Autodesk Inventor part; units mm, degrees
ref_plane "YZ Plane" through (0, 0, 0) normal (1, 0, 0) x (0, 1, 0)
ref_plane "XZ Plane" through (0, 0, 0) normal (0, 1, 0) x (-1, 0, 0)
ref_plane "XY Plane" through (0, 0, 0) normal (0, 0, 1) x (1, 0, 0)
sketch "Sketch1" plane through (0, 0, 0) normal (1, 0, 0) x (0, 1, 0)
  line L0 (0, 0) -> (60, 0)
  line L1 (60, 0) -> (60, 20)
  line L2 (60, 20) -> (0, 20)
  line L3 (0, 20) -> (0, 0)
  line L4 (60, 10) -> (0, 10) construction
  line L5 (60, 10) -> (30, 10) construction
  line L6 (30, 10) -> (0, 10) construction
  circle A0 centre (45, 10) radius 2.75
  circle A1 centre (15, 10) radius 2.75
  dimension "d0" = 60
  dimension "d1" = 20
  dimension "d2" = 5.5
  dimension "d3" = 5.5
extrude "Extrusion1" add sketch "Sketch1" against normal blind 6
sketch "Sketch2" plane through (-6, 0, 0) normal (-1, 0, 0) x (0, 0, 1)
  circle A0 centre (10, 45) radius 2.75
  circle A1 centre (10, 15) radius 2.75
  circle A2 centre (10, 45) radius 6.25
  circle A3 centre (10, 15) radius 6.25
  line L0 (20, 60) -> (0, 60)
  line L1 (12, 60) -> (12, 0)
  line L2 (8, 60) -> (8, 0)
  line L3 (0, 0) -> (20, 0)
  line L4 (0, 60) -> (0, 0)
  line L5 (20, 0) -> (20, 60)
  line L6 (12, 56.5) -> (17, 56.5)
  line L7 (17, 56.5) -> (17, 60)
  line L8 (8, 56.5) -> (3, 56.5)
  line L9 (3, 56.5) -> (3, 60)
  line L10 (8, 3.5) -> (3, 3.5)
  line L11 (3, 3.5) -> (3, 0)
  line L12 (12, 3.5) -> (17, 3.5)
  line L13 (17, 3.5) -> (17, 0)
  point P0 (12, 39.0786)
  point P1 (12, 50.9214)
  point P2 (8, 50.9214)
  point P3 (8, 39.0786)
  point P4 (8, 20.9214)
  point P5 (8, 9.0786)
  point P6 (12, 9.0786)
  point P7 (12, 20.9214)
  dimension "d6" = 3.5
  dimension "d7" = 8
  dimension "d8" = 8
  dimension "d9" = 3.5
  dimension "d10" = 3.5
  dimension "d11" = 3.5
  dimension "d16" = 3.5
extrude "Extrusion2" add sketch "Sketch2" along normal blind 22.1 contours A0 L1 A2 | A0 L2 A2 L1 | L1 A2 L2 A0 | A0 L2 A2 | A2 L2 L0 L1 | L1 A3 L2 A2 | A2 L2 A3 L10 L11 L3 L4 L0 L9 L8 | L1 L0 L7 L6 | L1 A1 L2 A3 | A3 L1 A1 | L8 L9 L0 L2 | L2 A1 A3 | L2 A1 L1 A3 | A3 L1 L3 L2 | L2 L3 L11 L10 | L12 L13 L3 L1
sketch "Sketch3" plane through (-28.1, 0, 0) normal (-1, 0, 0) x (0, 0, 1)
  circle A0 centre (10, 45) radius 2.75
  circle A1 centre (10, 15) radius 2.75
  line L0 (20, 0) -> (20, 60)
  line L1 (0, 0) -> (20, 0)
  line L2 (0, 0) -> (20, 0)
  line L3 (0, 0) -> (20, 0)
  line L4 (0, 60) -> (0, 0)
  line L5 (20, 60) -> (17, 60)
  line L6 (20, 60) -> (0, 60)
  line L7 (20, 60) -> (17, 60)
  point P0 (17, 0)
  point P1 (3, 0)
  point P2 (3, 60)
extrude "Extrusion3" add sketch "Sketch3" along normal blind 6
sketch "Sketch4" plane through (0, 0, 0) normal (0, 0, -1) x (-1, 0, 0)
  line L0 (0, 60) -> (0, 0)
  line L1 (34.1, 60) -> (34.1, 0)
  line L2 (0, 60) -> (34.1, 60)
  line L3 (34.1, 60) -> (34.1, 24.6)
  line L4 (34.1, 24.6) -> (0, 24.6)
  line L5 (0, 24.6) -> (0, 60)
  line L6 (34.1, 0) -> (34.1, 60)
  line L7 (0, 0) -> (0, 60)
  line L8 (34.1, 62.55) -> (0, 62.55)
  line L9 (0, 62.55) -> (0, 22.05)
  line L10 (0, 22.05) -> (34.1, 22.05)
  line L11 (34.1, 22.05) -> (34.1, 62.55)
  line L12 (0, 66.55) -> (34.1, 66.55)
  line L13 (34.1, 18.05) -> (0, 18.05)
  line L14 (2.6912, 62.55) -> (2.6912, 22.05) construction
  line L15 (34.1, 62.55) -> (34.1, 66.55)
  line L16 (0, 62.55) -> (0, 66.55)
  point P0 (34.1, 54.55)
  point P1 (0, 54.55)
  point P2 (2.6912, 42.3)
  dimension "d17" = 35.4
  dimension "d18" = 40.5
  dimension "d20" = 4
  dimension "d45" = 17.7
  dimension "d46" = 4
extrude "Extrusion4" add sketch "Sketch4" along normal blind 7.847
sketch "Sketch5" plane through (0, 0, -7.847) normal (0, 0, -1) x (-1, 0, 0)
  line L0 (34.1, 18.05) -> (34.1, 66.55)
  line L1 (34.1, 66.55) -> (0, 66.55)
  line L2 (0, 66.55) -> (0, 18.05)
  line L3 (0, 18.05) -> (34.1, 18.05)
  line L4 (34.1, 18.05) -> (34.1, 54.55)
  line L5 (0, 54.55) -> (0, 18.05)
  line L6 (34.1, 62.55) -> (0, 62.55)
  line L7 (0, 62.55) -> (0, 22.05)
  line L8 (0, 22.05) -> (34.1, 22.05)
  line L9 (34.1, 22.05) -> (34.1, 62.55)
  point P0 (0, 0)
  point P1 (0, 62.55)
  point P2 (34.1, 22.05)
  dimension "d23" = 40.5
  dimension "d24" = 4
extrude "Extrusion5" add sketch "Sketch5" along normal blind 7.28 contours L3 L2 L8 L0 | L6 L2 L1 L0
sketch "Sketch6" plane through (0, 0, 0) normal (1, 0, 0) x (0, 0, -1)
  line L0 (7.847, 22.05) -> (15.127, 22.05) construction
  line L1 (7.847, 62.55) -> (15.127, 62.55) construction
  line L2 (7.847, 22.05) -> (10.847, 22.05) construction
  line L3 (10.847, 22.05) -> (10.847, 62.55) construction
  line L4 (10.847, 62.55) -> (7.847, 62.55) construction
  line L5 (7.847, 62.55) -> (7.847, 22.05) construction
  line L6 (7.847, 22.05) -> (7.847, 62.55) construction
  line L7 (7.847, 42.3) -> (1.4795, 42.3) construction
  circle A0 centre (6.347, 42.3) radius 2.5 construction
  circle A1 centre (6.347, 42.3) radius 4.5
  line L8 (0, 60) -> (-20, 60)
  line L9 (-20, 60) -> (-20, 0)
  line L10 (-20, 0) -> (0, 0)
  line L11 (0, 0) -> (0, 18.05)
  circle A2 centre (-10, 45) radius 2.75
  circle A3 centre (-10, 15) radius 2.75
  circle A4 centre (6.347, 42.3) radius 5
  line L12 (0, 18.05) -> (15.127, 18.05)
  line L13 (15.127, 22.05) -> (15.127, 18.05)
  line L14 (7.847, 22.05) -> (15.127, 22.05)
  line L15 (7.847, 62.55) -> (7.847, 22.05)
  line L16 (7.847, 62.55) -> (15.127, 62.55)
  line L17 (15.127, 66.55) -> (15.127, 62.55)
  line L18 (0, 66.55) -> (15.127, 66.55)
  line L19 (0, 66.55) -> (0, 60)
  point P0 (7.847, 47.0697)
  point P1 (7.847, 37.5303)
  dimension "d27" = 3
  dimension "d28" = 5
  dimension "d29" = 2
  dimension "d30" = 2
  dimension "d31" = 0.5
extrude "Extrusion6" cut sketch "Sketch6" against normal through all contours L15 A1 | A1 L15 A4 picked at (4.8498, 43.4746) picked at (1.5593, 41.9128)
sketch "Sketch8" plane through (-34.1, 0, 0) normal (-1, 0, 0) x (0, 0, 1)
  line L0 (0, 18.05) -> (0, 0)
  line L1 (0, 0) -> (20, 0)
  line L2 (20, 0) -> (20, 60)
  line L3 (20, 60) -> (0, 60)
  circle A0 centre (10, 45) radius 2.75
  circle A1 centre (10, 15) radius 2.75
  line L4 (-0.2, 66.55) -> (-0.2, 18.05)
  line L5 (0, 18.05) -> (-15.127, 18.05)
  line L6 (0, 60) -> (0, 66.55)
  line L7 (0, 66.55) -> (-15.127, 66.55)
  line L8 (-15.127, 62.55) -> (-15.127, 66.55)
  line L9 (-7.847, 62.55) -> (-15.127, 62.55)
  line L10 (-7.847, 22.05) -> (-7.847, 37.5303)
  line L11 (-7.847, 22.05) -> (-15.127, 22.05)
  line L12 (-15.127, 18.05) -> (-15.127, 22.05)
  line L13 (0, 18.05) -> (-15.127, 18.05)
  arc A2 (-7.847, 37.5303) -> (-7.847, 47.0697) centre (-6.347, 42.3) ccw
  arc A3 (-7.847, 37.5303) -> (-7.847, 47.0697) centre (-6.347, 42.3) ccw
  line L14 (-7.847, 47.0697) -> (-7.847, 62.55)
  dimension "d34" = 0.2
extrude "Extrusion7" add sketch "Sketch8" along normal blind 17 contours L5 L12 L11 L10 A2 L14 L9 L8 L7 L4
sketch "Sketch9" plane through (-51.1, 0, 0) normal (-1, 0, 0) x (0, 0, 1)
  line L0 (-15.127, 22.05) -> (-15.127, 18.05)
  line L1 (-0.2, 18.05) -> (-0.2, 66.55)
  line L2 (-15.127, 22.05) -> (-15.127, 18.05)
  line L3 (-15.127, 18.05) -> (-15.127, 62.55)
  line L4 (-15.127, 62.55) -> (-7.847, 62.55)
  line L5 (-7.847, 37.5303) -> (-7.847, 22.05)
  line L6 (-7.847, 22.05) -> (-15.127, 22.05)
  line L7 (-15.127, 18.05) -> (-0.2, 18.05)
  line L8 (-0.2, 66.55) -> (-15.127, 66.55)
  line L9 (-15.127, 66.55) -> (-15.127, 62.55)
  arc A0 (-7.847, 37.5303) -> (-7.847, 47.0697) centre (-6.347, 42.3) ccw
  line L10 (-7.847, 62.55) -> (-7.847, 47.0697)
  point P0 (0, 0)
  point P1 (-15.127, 22.05)
extrude "Extrusion8" add sketch "Sketch9" along normal blind 5
sketch "Sketch10" plane through (-56.1, 0, 0) normal (-1, 0, 0) x (0, 0, 1)
  arc A0 (-7.847, 37.5303) -> (-7.847, 47.0697) centre (-6.347, 42.3) ccw
  circle A1 centre (-6.347, 42.3) radius 2.6
  point P0 (0, 0)
  dimension "d39" = 5.2
extrude "Extrusion9" cut sketch "Sketch10" against normal up to next
chamfer "Chamfer1" distance 3 angle 45 2 edges at (-56.1, 66.55, -7.6635) (-56.1, 18.05, -7.6635)
equation "\"d3\" = d2"
equation "\"d16\" = d6"
equation "\"d46\" = d20"
properties part number "Y Axis Belt Adjustable and Plate Spacer"
Design review of the part built by this model. Coordinates are the model's own, in mm. A direction names the side the tool comes from. Coordinates: 2 decimals unless noted, no trailing zeros. Loops run counter-clockwise (first coordinate to the right, second up) from the corner with the lowest first, then second, coordinate; pieces in that order, holes last. Notation, with made-up numbers: (27, 57.5) -> (75, 57.5) arc R24 ccw to (75, 70.5) -> close; hole circle Ø2 at (21, -20.5). An arc over 180 degrees is marked (long way). Use a Markdown table: item, result. Add a question column.
Item 1: We need section B-B, the plane y = 43.5. Write out the cut boundary in (x, z), and give its area (3 significant figures).
Item 2: We need section C-C, the plane y = 52.5. Write out the cut boundary in (x, z), and give its area (3 significant figures).
Item 3: We need section A-A, the plane x = -49. Write out the cut boundary in (y, z), and give its area (3 significant figures).
Item 4: Wall thickness on L1, parallel to Y at x = -12, z = -11; L2, parallel to X at y = 39.5, z = 18; L3, parallel to Y at x = -3, z = 2: over which ranges is each line inside the solid? List them lowest first. Write a range as from..to.
Item 5: Clearance check with flat-ended pins moving along their axes: P1, Ø12.5, axis at x = -36, y = 27, coming from the -Z side; P2, Ø7.5, axis at x = -38, z = -11.5, coming from the -Y side; P3, Ø4, axis at x = -24.5, y = 58.5, coming from the +Z side; P4, Ø7, axis at y = 45, z = 10, coming from the -X side. State where each tip first meets the part, or that it passes through.
Item 6: The part is to be moulded in two halves that separate along X. For faces 6 (the flat face through (-3, 30, 20)), 7 (the flat face through (-17, 54, 12)), 8 (the flat face through (-34.1, 34, 10)), say which applies: +X half, -X half, draft (parallel to the pull), parting line (faces both ways), or undercut.
Item 7: Machinability: for faces 1 (the flat face through (-17, 60, 10)), 2 (the flat face through (-56.1, 42.6, -9.4)), 3 (the flat face through (-17, 9, 0)), 4 (the cylindrical face through (-16.9, 15.11, 16.25)), 5 (the flat face through (-25, 22.05, -11)), which of the approach directions +Z, -Z, +X, -X, +Y, -Y give a long, thin tool a straight path to every point of the face, cutting with its end or side? Answer none if there is none.
Numbers:
| question | item | result |
|---|---|---|
| 1 | outline | (-56.1, -15.13) -> (-51.1, -15.13) -> (-51.1, -8.65) -> (-56.1, -8.65) -> close; (-56.1, -4.04) -> (-51.1, -4.04) -> (-51.1, -1.49) -> (0, -1.49) -> (0, 7.7) -> (-34.1, 7.7) -> (-34.1, -0.2) -> (-56.1, -0.2) -> close; (-34.1, 12.3) -> (0, 12.3) -> (0, 20) -> (-6, 20) -> (-6, 16.07) -> (-28.1, 16.07) -> (-28.1, 20) -> (-34.1, 20) -> close |
| 1 | area | 562 mm^2 |
| 2 | outline | (-56.1, -15.13) -> (-51.1, -15.13) -> (-51.1, -7.85) -> (0, -7.85) -> (0, 20) -> (-6, 20) -> (-6, 12) -> (-28.1, 12) -> (-28.1, 20) -> (-34.1, 20) -> (-34.1, -0.2) -> (-56.1, -0.2) -> close |
| 2 | area | 977 mm^2 |
| 3 | outline | (18.05, -15.13) -> (22.05, -15.13) -> (22.05, -7.85) -> (37.53, -7.85) arc R5 cw (long way) to (47.07, -7.85) -> (62.55, -7.85) -> (62.55, -15.13) -> (66.55, -15.13) -> (66.55, -0.2) -> (18.05, -0.2) -> close |
| 3 | area | 375 mm^2 |
| 4 | L1 | y = 18.05..22.05, 62.55..66.55 |
| 4 | L2 | x = -34.1..-28.1, -6..0 |
| 4 | L3 | y = 0..60 |
| 5 | P1 | stops at z = -15.13 |
| 5 | P2 | stops at y = 18.05 |
| 5 | P3 | stops at z = 17 |
| 5 | P4 | stops at x = -34.1 |
| 6 | face 6 | draft |
| 6 | face 7 | undercut |
| 6 | face 8 | -X half |
| 7 | face 1 | +Z, +X, -X, +Y |
| 7 | face 2 | +Z, -Z, -X, +Y, -Y |
| 7 | face 3 | -Z, +X, -X, -Y |
| 7 | face 4 | +Z |
| 7 | face 5 | -Z, +X |
